```python
from build123d import *

# Parameters (mm, degrees)
SKETCH1_W           = 280
SKETCH1_H           = 140
BOSS_EXTRUDE1_DEPTH = 10
FILLET1_R           = 14
SKETCH2_R           = 25
CUT_EXTRUDE1_DEPTH  = 10


with BuildPart() as part:
    # Sketch1 → Boss-Extrude1 (new body)
    with BuildSketch(Plane(origin=(0, 0, 0), x_dir=(1, 0, 0), z_dir=(0, 1, 0))):
        Rectangle(SKETCH1_W, SKETCH1_H)
    extrude(amount=BOSS_EXTRUDE1_DEPTH)

    # Fillet1
    fillet1_edges = [part.edges().sort_by_distance(p)[0] for p in [
        (140, 5, 70),
        (-140, 5, 70),
    ]]
    fillet(fillet1_edges, radius=FILLET1_R)

    # Sketch2 → Cut-Extrude1 (cut)
    with BuildSketch(Plane(origin=(0, 10, 0), x_dir=(1, 0, 0), z_dir=(0, 1, 0))):
        with Locations(Location((0, 0, 0), (0, 0, 270))):
            Circle(SKETCH2_R)
    extrude(amount=-CUT_EXTRUDE1_DEPTH, mode=Mode.SUBTRACT)


solid = part.part
```
Check sheet for the modelled part. Datum: model origin and axes. Units: mm. Coordinates: 2 decimals unless noted, no trailing zeros. Order: outer loops, then holes, each group sorted by start corner. A loop starts at its lowest first (then second) coordinate and runs counter-clockwise, first axis right, second up. Notation, with made-up numbers: (64.5, 16) -> (73.5, 16) arc R25 ccw to (73.5, 55) -> close; hole circle Ø10 at (36.5, -0.5). An arc over 180 degrees is marked (long way). Write item = value, one per line. Start each with the question number.
1) Cross-section at A-A (x = 0). Enter the section's corners in (y, z).
2) Cross-section at B-B (y = 1.75). Enter the section's corners in (x, z).
3) Mould release check, pull along X, two halves, no side actions. Record for faces 1 (the cylindrical face through (7.509, 5.07, 23.846)), 2 (the cylindrical face through (135.8, 5.1, 66)), 3 (the flat face through (-2, 5, 70)), 4 (the cylindrical face through (-136, 5.1, 65.8)): +X half, -X half, draft (parallel to the pull), parting line (faces both ways), or undercut.
4) Material ranges on L1, parallel to X at y = 3.5, z = 0; L2, parallel to X at y = 4.25, z = 5; L3, parallel to Z at x = 20.5, y = 6, recorded low to high.
5) Cross-section at C-C (z = 0). Enter the section's corners in (x, y).
Ans:
q1.outline = (0, -70) -> (10, -70) -> (10, -25) -> (0, -25) -> close; (0, 25) -> (10, 25) -> (10, 70) -> (0, 70) -> close
q2.outline = (-140, -70) -> (140, -70) -> (140, 56) arc R14 ccw to (126, 70) -> (-126, 70) arc R14 ccw to (-140, 56) -> close; hole circle Ø50 at (0, 0)
q3.face_1 = undercut
q3.face_2 = +X half
q3.face_3 = draft
q3.face_4 = -X half
q4.L1 = -140 to -25, 25 to 140
q4.L2 = -140 to -24.49, 24.49 to 140
q4.L3 = -70 to -14.31, 14.31 to 70
q5.outline = (-140, 0) -> (-25, 0) -> (-25, 10) -> (-140, 10) -> close; (25, 0) -> (140, 0) -> (140, 10) -> (25, 10) -> close
